Geometry check sheet. Reference: the model listing, model coordinates, mm. Face numbers are marked on the shaded views. A direction names the side the tool comes from. Round coordinates to 2 decimals unless told otherwise and drop trailing zeros. Write each loop counter-clockwise with the first axis right and the second up, starting at its lowest first coordinate (ties: lowest second). Pieces come first, ordered by that corner, then holes. Notation, with made-up numbers: (59, 22) -> (90, 22) arc R32 ccw to (90, 52) -> close; hole circle Ø5 at (-26.75, -13.75). An arc over 180 degrees is marked (long way). One line per question, with ' | ' between items.
```python
from build123d import *

# Parameters (mm, degrees)
SKETCH1_W                                       = 156.21
SKETCH1_H                                       = 25.4
BOSS_EXTRUDE1_DEPTH                             = 5.08
BOSS_EXTRUDE1_2_DEPTH                           = 5.08
SKETCH1_3_W                                     = 156.21
SKETCH1_3_H                                     = 121.92
SKETCH1_3_W_2                                   = 146.05
SKETCH1_3_H_2                                   = 53.34
BOSS_EXTRUDE2_DEPTH                             = 63.5
SKETCH2_W                                       = 156.21
SKETCH2_H                                       = 121.92
BOSS_EXTRUDE3_DEPTH                             = 5.08
SKETCH3_W                                       = 20.32
SKETCH3_H                                       = 20.32
CUT_EXTRUDE1_DEPTH                              = 5.08
CBORE_FOR_10_SOCKET_HEAD_CAP_SCREW1_D           = 5.6134
CBORE_FOR_10_SOCKET_HEAD_CAP_SCREW1_CBORE_D     = 9.525
CBORE_FOR_10_SOCKET_HEAD_CAP_SCREW1_CBORE_DEPTH = 4.826
CBORE_FOR_10_SOCKET_HEAD_CAP_SCREW2_D           = 5.6134
CBORE_FOR_10_SOCKET_HEAD_CAP_SCREW2_CBORE_D     = 9.525
CBORE_FOR_10_SOCKET_HEAD_CAP_SCREW2_CBORE_DEPTH = 4.826


with BuildPart() as part:
    # Sketch1 → Boss-Extrude1 (new body)
    with BuildSketch(Plane(origin=(0, 0, 0), x_dir=(0, 0, -1), z_dir=(1, 0, 0))):
        with Locations((0, 73.66)):
            Rectangle(SKETCH1_W, SKETCH1_H)
    extrude(amount=BOSS_EXTRUDE1_DEPTH)



with BuildPart() as body_2:
    # Sketch1 → Boss-Extrude1 2 (new body)
    with BuildSketch(Plane(origin=(0, 0, 0), x_dir=(0, 0, -1), z_dir=(1, 0, 0))):
        with Locations((0, -73.66)):
            Rectangle(SKETCH1_W, SKETCH1_H)
    extrude(amount=BOSS_EXTRUDE1_2_DEPTH)


with BuildPart() as part_1:
    add(part.part)

    add(body_2.part)  # Boss-Extrude2 merges body 2
    # Sketch1<3> → Boss-Extrude2 (add)
    with BuildSketch(Plane(origin=(0, 0, 0), x_dir=(0, 0, -1), z_dir=(1, 0, 0))):
        Rectangle(SKETCH1_3_W, SKETCH1_3_H)
        with Locations((0, -29.21)):
            Rectangle(SKETCH1_3_W_2, SKETCH1_3_H_2, mode=Mode.SUBTRACT)
        with Locations((0, 29.21)):
            Rectangle(SKETCH1_3_W_2, SKETCH1_3_H_2, mode=Mode.SUBTRACT)
    extrude(amount=BOSS_EXTRUDE2_DEPTH)

    # Sketch2 → Boss-Extrude3 (add)
    with BuildSketch(Plane(origin=(63.5, 0, 0), x_dir=(0, 0, -1), z_dir=(1, 0, 0))):
        Rectangle(SKETCH2_W, SKETCH2_H)
    extrude(amount=BOSS_EXTRUDE3_DEPTH)

    # Sketch3 → Cut-Extrude1 (cut)
    with BuildSketch(Plane.XY.offset(78.105)):
        with Locations((36.83, 33.02)):
            Rectangle(SKETCH3_W, SKETCH3_H)
        with Locations((36.83, -33.02)):
            Rectangle(SKETCH3_W, SKETCH3_H)
    extrude(amount=-CUT_EXTRUDE1_DEPTH, mode=Mode.SUBTRACT)

    # CBORE for #10 Socket Head Cap Screw1 (through all)
    with Locations(Plane(origin=(5.08, 0, 0), x_dir=(0, 0, -1), z_dir=(1, 0, 0))):
        with Locations((0, 73.66), (-56.783367635, 73.66), (57.284766025, 73.66)):
            CounterBoreHole(CBORE_FOR_10_SOCKET_HEAD_CAP_SCREW1_D / 2, CBORE_FOR_10_SOCKET_HEAD_CAP_SCREW1_CBORE_D / 2, CBORE_FOR_10_SOCKET_HEAD_CAP_SCREW1_CBORE_DEPTH)

    # CBORE for #10 Socket Head Cap Screw2 (through all)
    with Locations(Plane(origin=(5.08, 0, 0), x_dir=(0, 0, -1), z_dir=(1, 0, 0))):
        with Locations((0, -73.66), (-57.53546522, -73.66), (59.541058779, -73.66)):
            CounterBoreHole(CBORE_FOR_10_SOCKET_HEAD_CAP_SCREW2_D / 2, CBORE_FOR_10_SOCKET_HEAD_CAP_SCREW2_CBORE_D / 2, CBORE_FOR_10_SOCKET_HEAD_CAP_SCREW2_CBORE_DEPTH)


solid = part_1.part
```
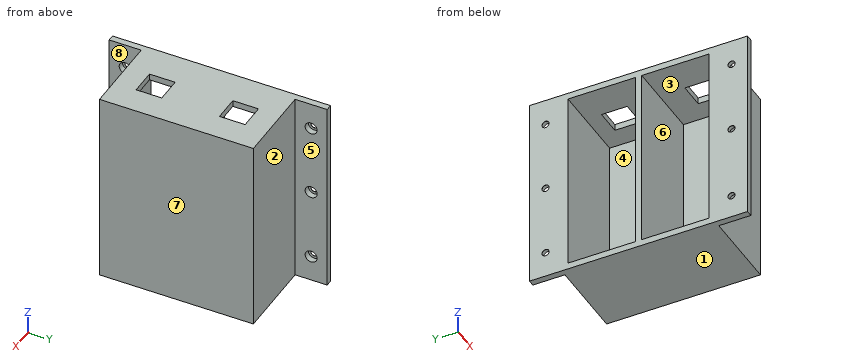
(1) Draft check along Y on the marked faces 1, 2, 3 and 4. Enter one of: +Y half, -Y half, draft (parallel to the pull), parting line (faces both ways), or undercut.
Resolved:
face 1: draft | face 2: +Y half | face 3: undercut | face 4: undercut
(2) Material ranges on line 1 (Y direction, x = 18.5, z = 61); line 2 (Y direction, x = 3.1, z = 0); line 3 (Z direction, x = 24, y = -7.5) (3 decimals), recorded low to high.
Resolved:
line 1: y = -60.96 to -55.88, -2.54 to 2.54, 55.88 to 60.96 | line 2: y = -86.36 to -78.42, -68.9 to -55.88, -2.54 to 2.54, 55.88 to 68.9, 78.42 to 86.36 | line 3: z = -78.105 to -73.025, 73.025 to 78.105
(3) Sectioned sample at B-B on z = 0. Count the separate pieces of the cut face and the enclosed holes in it, then the cut area to 3 significant figures.
Resolved:
separate pieces: 3 | enclosed holes: 0 | area: 1,750 mm2
(4) Sectioned sample at A-A on y = -35.5. Record the cut outline in (x, z) (3 decimals), then the cut area to 3 significant figures.
Resolved:
outline: (0, -78.105) -> (68.58, -78.105) -> (68.58, 78.105) -> (46.99, 78.105) -> (46.99, 73.025) -> (63.5, 73.025) -> (63.5, -73.025) -> (0, -73.025) -> close; (0, 73.025) -> (26.67, 73.025) -> (26.67, 78.105) -> (0, 78.105) -> close | area: 1,340 mm2
(5) Access from +Z, -Z, +X, -X, +Y, -Y to the whole of each face (thin tool, end or side, straight path). Record for the marked faces 5, 6, 7 and 8.
Resolved:
face 5: +Z, -Z, +X, +Y | face 6: -X | face 7: +Z, -Z, +X, +Y, -Y | face 8: +Z, -Z, +X, -Y
(6) Sectioned sample at D-D on x = 50.5. Record the cut outline in (y, z) (3 decimals), then the cut area to 3 significant figures.
Resolved:
outline: (-60.96, -78.105) -> (60.96, -78.105) -> (60.96, 78.105) -> (-60.96, 78.105) -> close; hole (-55.88, -73.025) -> (-2.54, -73.025) -> (-2.54, 73.025) -> (-55.88, 73.025) -> close; hole (2.54, -73.025) -> (55.88, -73.025) -> (55.88, 73.025) -> (2.54, 73.025) -> close | area: 3,460 mm2
(7) Go/stop test with flat-tipped pins: pin 1 (6.5 mm diameter, centred on y = -73.66, z = 0, fed in from -X); pin 2 (2 mm diameter, centred on x = 11, z = -1, fed in from +Y); pin 3 (7.5 mm diameter, centred on y = -73.66, z = 57.54, fed in from +X); pin 4 (3 mm diameter, centred on y = 18.5, z = -55.5, fed in from -X). Record where each tip stops, or that it passes through.
Resolved:
pin 1: stops at x = 0 | pin 2: stops at y = 60.96 | pin 3: stops at x = 0.25 | pin 4: stops at x = 63.5
